Autodesk Inventor part; units mm, degrees
ref_plane "YZ Plane" through (0, 0, 0) normal (1, 0, 0) x (0, 1, 0)
ref_plane "XZ Plane" through (0, 0, 0) normal (0, 1, 0) x (-1, 0, 0)
ref_plane "XY Plane" through (0, 0, 0) normal (0, 0, 1) x (1, 0, 0)
sketch "Sketch1" plane through (0, 0, 0) normal (0, 0, 1) x (1, 0, 0)
  line L0 (-59, 61.875) -> (-59, 100)
  line L1 (-34, -100) -> (-54, -100)
  line L2 (-14, -12.375) -> (-8, -12.375)
  line L3 (-8, 37.125) -> (-14, 37.125)
  line L4 (-14, 61.875) -> (-8, 61.875)
  line L5 (-8, 12.375) -> (-14, 12.375)
  line L6 (-8, -37.125) -> (-14, -37.125)
  line L7 (-14, -61.875) -> (-8, -61.875)
  line L8 (-14, 61.875) -> (-14, 100)
  line L9 (-14, 37.125) -> (-14, 12.375)
  line L10 (-8, 37.125) -> (-8, 61.875)
  line L11 (-14, -12.375) -> (-14, -37.125)
  line L12 (-8, -61.875) -> (-8, -37.125)
  line L13 (-8, -12.375) -> (-8, 12.375)
  line L14 (-14, -61.875) -> (-14, -100)
  line L15 (-14, -100) -> (-59, -100)
  line L16 (-14, 100) -> (-14, 102)
  line L17 (-14, 102) -> (-59, 102)
  line L18 (-59, 102) -> (-59, 100)
  line L19 (-59, 61.875) -> (-59, -100)
  point P0 (-60, 61.875)
  point P1 (-60, 37.125)
  point P2 (-60, 12.375)
  point P3 (-60, -12.375)
  point P4 (-60, -37.125)
  point P5 (-60, -61.875)
  dimension "d23" = 45
extrude "Extrusion1" add sketch "Sketch1" along normal blind 6
properties part number "Side_2"
Can you work these out from the model? Positions are in its coordinate system, mm. A direction names the side the tool comes from. Give positions to 0.01 mm unless a question says otherwise; leave off trailing zeros. Loops run counter-clockwise (first coordinate to the right, second up) from the corner with the lowest first, then second, coordinate; pieces in that order, holes last. Notation, with made-up numbers: (13.25, 52.25) - (61.25, 52.25) arc R34 ccw to (61.25, 90.25) - close; hole circle Ø5 at (79.25, 69). An arc over 180 degrees is marked (long way). Answer as a JSON object with one key per item and string values.
Q1. Which directions (+Z, -Z, +X, -X, +Y, -Y) give clear straight access to the entire face, cutting with the end or side of a thin tool? Please do faces 5 (the flat face through (-14, -81, 3)), 6 (the flat face through (-14, 82, 3)), 7 (the flat face through (-34, 2, 6)), 8 (the flat face through (-14, 25, 3)).
Geometry says:
{"face 5": "+Z, -Z, +X, -Y", "face 6": "+Z, -Z, +X, +Y", "face 7": "+Z, +X, -X, +Y, -Y", "face 8": "+Z, -Z, +X"}
Q2. Imagine slicing it at A-A on z = 4.5. Write out the boundary of the cut face in (x, y) (3 decimals).
Geometry says:
{"outline": "(-59, -100) - (-14, -100) - (-14, -61.875) - (-8, -61.875) - (-8, -37.125) - (-14, -37.125) - (-14, -12.375) - (-8, -12.375) - (-8, 12.375) - (-14, 12.375) - (-14, 37.125) - (-8, 37.125) - (-8, 61.875) - (-14, 61.875) - (-14, 102) - (-59, 102) - close"}
Q3. Will these pins go through, and if not, where does the flat tip stop? P1, Ø1.8, axis at x = -11, z = 3.5, coming from the -Y side (3 decimals); P2, Ø1.8, axis at y = 75.5, z = 2.5, coming from the +X side; P3, Ø1.8, axis at x = -12, z = 4.5, coming from the +Y side (3 decimals).
Geometry says:
{"P1": "y = -61.875", "P2": "x = -14", "P3": "y = 61.875"}
Q4. Imagine slicing it at B-B on y = -67.5. Write out the boundary of the cut face in (x, z).
Geometry says:
{"outline": "(-59, 0) - (-14, 0) - (-14, 6) - (-59, 6) - close"}
Q5. If we mould it in two halves opening along Y, with no side actions, what happens to faces 1 (the flat face through (-11, -37.125, 3)), 2 (the flat face through (-11, 61.875, 3)), 3 (the flat face through (-11, -12.375, 3)), 4 (the flat face through (-34, 2, 0))? For each: pulls with the +Y half, pulls with the -Y half, needs draft (parallel to the pull), parting line crosses it, or undercut.
Geometry says:
{"face 1": "undercut", "face 2": "pulls with the +Y half", "face 3": "undercut", "face 4": "needs draft"}
Q6. If I drill on L1, parallel to X at y = 62, z = 5.15, over which ranges is the centre line in solid material (lowest first)?
Geometry says:
{"L1": "-59 to -14"}
